Autodesk Inventor part; units mm, degrees
ref_plane "YZ Plane" through (0, 0, 0) normal (1, 0, 0) x (0, 1, 0)
ref_plane "XZ Plane" through (0, 0, 0) normal (0, 1, 0) x (-1, 0, 0)
ref_plane "XY Plane" through (0, 0, 0) normal (0, 0, 1) x (1, 0, 0)
sketch "Sketch1" plane through (0, 0, 0) normal (0, 1, 0) x (-1, 0, 0)
  line L0 (0, 0) -> (-101.6, 0) construction
  line L1 (-101.6, 0) -> (-101.6, -101.6) construction
  line L2 (-101.6, -101.6) -> (0, -101.6) construction
  line L3 (0, -101.6) -> (0, 0) construction
  line L4 (-101.6, 15.5049) -> (-81.6, 15.5049) construction
  line L5 (-81.6, 15.5049) -> (-81.6, -123.9701) construction
  line L6 (-81.6, -123.9701) -> (-101.6, -123.9701) construction
  line L7 (-101.6, -123.9701) -> (-101.6, 15.5049) construction
  line L8 (-81.6, -101.6) -> (54.3539, 34.3539) construction
  line L9 (54.3539, 34.3539) -> (40.2117, 48.496) construction
  line L10 (40.2117, 48.496) -> (-81.6, -73.3157) construction
  line L11 (-101.6, -101.6) -> (-81.6, -101.6)
  line L12 (-81.6, -101.6) -> (-3.5401, -23.5401)
  line L13 (-8.0303, -12.7) -> (-101.6, -12.7)
  line L14 (-101.6, -12.7) -> (-101.6, -101.6)
  circle A0 centre (-66.2, -72.0579) radius 4.2211
  circle A1 centre (-28.1, -33.9579) radius 4.2211
  circle A2 centre (-91.6, -33.9579) radius 4.2211
  circle A3 centre (-91.6, -72.0579) radius 4.2211
  line L15 (-81.6, -101.6) -> (-101.6, -121.6)
  line L16 (-101.6, -101.6) -> (-101.6, -121.6)
  line L17 (-28.1, -33.9579) -> (-66.2, -72.0579) construction
  line L18 (-8.0303, -12.7) -> (7.3, -12.7)
  line L19 (-3.5401, -23.5401) -> (7.3, -12.7)
  circle A4 centre (-47.15, -53.0079) radius 3.9521
  circle A5 centre (-91.6, -53.0079) radius 4.2211
  dimension "d0" = 101.6
  dimension "d1" = 101.6
  dimension "d2" = 20
  dimension "d3" = 20
  dimension "d4" = 45
  dimension "d11" = 10
  dimension "d13" = 10
  dimension "d15" = 25.4
  dimension "d16" = 38.1
  dimension "d17" = 88.9
extrude "Extrusion1" add sketch "Sketch1" along normal blind 3.175 contours L14 L13 L18 L19 L12 L11 | A0 | A1 | A2 | A3 | A4 | A5
hole "Hole1" at (91.6, 0, -33.9579) at (91.6, 0, -72.0579) at (66.2, 0, -72.0579) at (28.1, 0, -33.9579) at (47.15, 0, -53.0079) at (91.6, 0, -53.0079) direction (0, 1, 0) diameter 5.5118 end through all
equation "\"d3\" = d2"
properties part number "CH-1-01-FrontKneeJoint"
Here's how the part is built. I have some questions about the finished solid (model axes, mm). Round coordinates to 2 decimals unless told otherwise and drop trailing zeros. Loops run counter-clockwise (first coordinate to the right, second up) from the corner with the lowest first, then second, coordinate; pieces in that order, holes last. Notation, with made-up numbers: (2, 86) - (22, 86) arc R27 cw to (22, 106) - close; hole circle Ø5 at (55.25, 66). An arc over 180 degrees is marked (long way). One line per question, with ' | ' between items. Start each with the question number.
Q1. I want a section at C-C (y = 0.8). Write out the boundary of the cut face in (x, z).
Q2. Please list where these lines run through material, in increasing order: line 1 (Z direction, x = 91.6, y = 1.1); line 2 (Z direction, x = 94, y = 0.95); line 3 (X direction, y = 3, z = -53.5). Write a range as [from, to].
Q3. We'd pull the mould along X, two halves only. Please class faces 1 (the cylindrical face through (46.322, 1.61, -55.637)), 2 (the flat face through (60, 0, -47)), 3 (the flat face through (38, 2, -58)): +X half, -X half, draft (parallel to the pull), parting line (faces both ways), or undercut.
Q4. Will this pin go through, and if not, where does the flat tip stop? pin 1 (5 mm diameter, centred on x = 91.6, z = -33.96, fed in from +Y).
Q5. I want a section at B-B (x = 91.6). Write out the boundary of the cut face in (y, z) (3 decimals).
Q6. I want a section at D-D (z = -34). Write out the boundary of the cut face in (x, y) (3 decimals), then the cut area to 3 significant figures.
Q7. I want a section at A-A (x = 66.2). Write out the boundary of the cut face in (y, z) (3 decimals), then the cut area to 3 significant figures.
Response values:
1) outline: (-7.3, -12.7) - (81.6, -101.6) - (101.6, -101.6) - (101.6, -12.7) - close; hole circle Ø5.51 at (28.1, -33.96); hole circle Ø5.51 at (47.15, -53.01); hole circle Ø5.51 at (66.2, -72.06); hole circle Ø5.51 at (91.6, -72.06); hole circle Ø5.51 at (91.6, -53.01); hole circle Ø5.51 at (91.6, -33.96)
2) line 1: z = [-101.6, -74.81], [-69.3, -55.76], [-50.25, -36.71], [-31.2, -12.7] | line 2: z = [-101.6, -73.41], [-70.7, -54.36], [-51.65, -35.31], [-32.6, -12.7] | line 3: x = [33.5, 44.44], [49.86, 88.89], [94.31, 101.6]
3) face 1: undercut | face 2: draft | face 3: -X half
4) pin 1: passes through
5) outline: (0, -101.6) - (3.175, -101.6) - (3.175, -74.814) - (0, -74.814) - close; (0, -69.302) - (3.175, -69.302) - (3.175, -55.764) - (0, -55.764) - close; (0, -50.252) - (3.175, -50.252) - (3.175, -36.714) - (0, -36.714) - close; (0, -31.202) - (3.175, -31.202) - (3.175, -12.7) - (0, -12.7) - close
6) outline: (14, 0) - (25.344, 0) - (25.344, 3.175) - (14, 3.175) - close; (30.856, 0) - (88.844, 0) - (88.844, 3.175) - (30.856, 3.175) - close; (94.356, 0) - (101.6, 0) - (101.6, 3.175) - (94.356, 3.175) - close | area: 243 mm²
7) outline: (0, -86.2) - (3.175, -86.2) - (3.175, -74.814) - (0, -74.814) - close; (0, -69.302) - (3.175, -69.302) - (3.175, -12.7) - (0, -12.7) - close | area: 216 mm²
